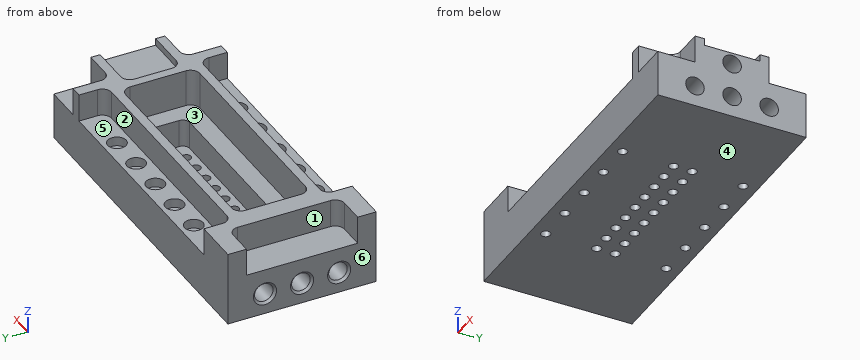
```python
from build123d import *

# Parameters (mm, degrees)
SKETCH1_W           = 230.1875
SKETCH1_H           = 101.6
BASE_EXTRUDE_DEPTH  = 50.8
CUT_EXTRUDE1_DEPTH  = 25.4
CUT_EXTRUDE2_DEPTH  = 19.05
CUT_EXTRUDE3_DEPTH  = 19.05
SKETCH5_R           = 6.35
CUT_EXTRUDE4_DEPTH  = 25.4
CHAMFER2_SIZE       = 1.5748
CUT_EXTRUDE5_START  = -25.4
SKETCH6_R           = 6.35
CUT_EXTRUDE5_DEPTH  = 25.4
CUT_EXTRUDE6_DEPTH  = 19.05
SKETCH8_R           = 3.175
CUT_EXTRUDE7_DEPTH  = 135.113217679
CUT_EXTRUDE8_DEPTH  = 19.05
SKETCH10_R          = 3.175
CUT_EXTRUDE9_DEPTH  = 131.455414438
SKETCH11_R          = 6.35
CUT_EXTRUDE10_DEPTH = 6.35
CUT_EXTRUDE11_DEPTH = 4.7498


with BuildPart() as part:
    # Sketch1 → Base-Extrude (new body)
    with BuildSketch(Plane.XY):
        with Locations((0.79375, 0)):
            Rectangle(SKETCH1_W, SKETCH1_H)
    extrude(amount=BASE_EXTRUDE_DEPTH)

    # Sketch2 → Cut-Extrude1 (cut)
    with BuildSketch(Plane.XY.offset(50.8)):
        with BuildLine():
            Line((-69.85, 25.4), (69.85, 25.4))
            ThreePointArc((69.85, 25.4), (74.340128061, 23.540128061), (76.2, 19.05))
            Line((76.2, 19.05), (76.2, -19.05))
            ThreePointArc((76.2, -19.05), (74.340128061, -23.540128061), (69.85, -25.4))
            Line((69.85, -25.4), (-69.85, -25.4))
            ThreePointArc((-69.85, -25.4), (-74.340128061, -23.540128061), (-76.2, -19.05))
            Line((-76.2, -19.05), (-76.2, 19.05))
            ThreePointArc((-76.2, 19.05), (-74.340128061, 23.540128061), (-69.85, 25.4))
        make_face()
    extrude(amount=-CUT_EXTRUDE1_DEPTH, mode=Mode.SUBTRACT)

    # Sketch3 → Cut-Extrude2 (cut)
    with BuildSketch(Plane.XY.offset(50.8)):
        with BuildLine():
            Line((136.525, 61.9125), (90.4875, 61.9125))
            Line((90.4875, 61.9125), (90.4875, 31.75))
            ThreePointArc((90.4875, 31.75), (92.347371939, 27.259871939), (96.8375, 25.4))
            Line((96.8375, 25.4), (136.525, 25.4))
            Line((136.525, 25.4), (136.525, 61.9125))
        make_face()
        with BuildLine():
            Line((136.525, -57.15), (90.4875, -57.15))
            Line((90.4875, -57.15), (90.4875, -31.75))
            ThreePointArc((90.4875, -31.75), (92.347371939, -27.259871939), (96.8375, -25.4))
            Line((96.8375, -25.4), (136.525, -25.4))
            Line((136.525, -25.4), (136.525, -57.15))
        make_face()
    extrude(amount=-CUT_EXTRUDE2_DEPTH, mode=Mode.SUBTRACT)

    # Sketch4 → Cut-Extrude3 (cut)
    with BuildSketch(Plane.XY.offset(50.8)):
        with BuildLine():
            Line((-120.65, 38.1), (-96.8375, 38.1))
            ThreePointArc((-96.8375, 38.1), (-92.347371939, 36.240128061), (-90.4875, 31.75))
            Line((-90.4875, 31.75), (-90.4875, -31.75))
            ThreePointArc((-90.4875, -31.75), (-92.347371939, -36.240128061), (-96.8375, -38.1))
            Line((-96.8375, -38.1), (-120.65, -38.1))
            Line((-120.65, -38.1), (-120.65, 38.1))
        make_face()
    extrude(amount=-CUT_EXTRUDE3_DEPTH, mode=Mode.SUBTRACT)

    # Sketch5 → Cut-Extrude4 (cut)
    with BuildSketch(Plane.ZY.offset(114.3)):
        with Locations((14.2875, 0)):
            Circle(SKETCH5_R)
        with Locations((14.2875, -25.4)):
            Circle(SKETCH5_R)
        with Locations((14.2875, 25.4)):
            Circle(SKETCH5_R)
    extrude(amount=-CUT_EXTRUDE4_DEPTH, mode=Mode.SUBTRACT)

    # Chamfer2
    chamfer2_edges = [part.edges().sort_by_distance(p)[0] for p in [
        (-114.3, -25.4, 7.9375),
        (-114.3, 0, 7.9375),
        (-114.3, 25.4, 7.9375),
    ]]
    chamfer(chamfer2_edges, length=CHAMFER2_SIZE)

    # Sketch6 → Cut-Extrude5 (cut)
    with BuildSketch(Plane(origin=(115.8875, 0, 0), x_dir=(0, 0, -1), z_dir=(1, 0, 0)).offset(CUT_EXTRUDE5_START)):
        with Locations((-38.1, 0)):
            Circle(SKETCH6_R)
        with Locations(Location((-14.2875, 0, 0), (0, 0, 180))):
            Circle(SKETCH6_R)
        with Locations(Location((-14.2875, 25.4, 0), (0, 0, 180))):
            Circle(SKETCH6_R)
        with Locations(Location((-14.2875, -25.4, 0), (0, 0, 180))):
            Circle(SKETCH6_R)
    extrude(amount=CUT_EXTRUDE5_DEPTH, mode=Mode.SUBTRACT)

    # Sketch7 → Cut-Extrude6 (cut)
    with BuildSketch(Plane.XY.offset(25.4)):
        with BuildLine():
            Line((-58.7375, 12.7), (58.7375, 12.7))
            ThreePointArc((58.7375, 12.7), (62.105096045, 11.305096045), (63.5, 7.9375))
            Line((63.5, 7.9375), (63.5, -7.9375))
            ThreePointArc((63.5, -7.9375), (62.105096045, -11.305096045), (58.7375, -12.7))
            Line((58.7375, -12.7), (-58.7375, -12.7))
            ThreePointArc((-58.7375, -12.7), (-62.105096045, -11.305096045), (-63.5, -7.9375))
            Line((-63.5, -7.9375), (-63.5, 7.9375))
            ThreePointArc((-63.5, 7.9375), (-62.105096045, 11.305096045), (-58.7375, 12.7))
        make_face()
    extrude(amount=-CUT_EXTRUDE6_DEPTH, mode=Mode.SUBTRACT)

    # Sketch8 → Cut-Extrude7 (cut, through all)
    with BuildSketch(Plane.XY.offset(6.35)):
        with Locations((-50.8, 6.35)):
            Circle(SKETCH8_R)
        with Locations((-38.1, 6.35)):
            Circle(SKETCH8_R)
        with Locations((-25.4, 6.35)):
            Circle(SKETCH8_R)
        with Locations((-12.7, 6.35)):
            Circle(SKETCH8_R)
        with Locations((0, 6.35)):
            Circle(SKETCH8_R)
        with Locations((12.7, 6.35)):
            Circle(SKETCH8_R)
        with Locations((25.4, 6.35)):
            Circle(SKETCH8_R)
        with Locations((38.1, 6.35)):
            Circle(SKETCH8_R)
        with Locations((50.8, 6.35)):
            Circle(SKETCH8_R)
        with Locations((-50.8, -6.35)):
            Circle(SKETCH8_R)
        with Locations((-38.1, -6.35)):
            Circle(SKETCH8_R)
        with Locations((-25.4, -6.35)):
            Circle(SKETCH8_R)
        with Locations((-12.7, -6.35)):
            Circle(SKETCH8_R)
        with Locations((0, -6.35)):
            Circle(SKETCH8_R)
        with Locations((12.7, -6.35)):
            Circle(SKETCH8_R)
        with Locations((25.4, -6.35)):
            Circle(SKETCH8_R)
        with Locations((38.1, -6.35)):
            Circle(SKETCH8_R)
        with Locations((50.8, -6.35)):
            Circle(SKETCH8_R)
    extrude(amount=-CUT_EXTRUDE7_DEPTH, mode=Mode.SUBTRACT)

    # Sketch9 → Cut-Extrude8 (cut)
    with BuildSketch(Plane.XY.offset(50.8)):
        with BuildLine():
            Line((-82.55, 63.5), (82.55, 63.5))
            Line((82.55, 63.5), (82.55, 38.1))
            ThreePointArc((82.55, 38.1), (80.690128061, 33.609871939), (76.2, 31.75))
            Line((76.2, 31.75), (-76.2, 31.75))
            ThreePointArc((-76.2, 31.75), (-80.690128061, 33.609871939), (-82.55, 38.1))
            Line((-82.55, 38.1), (-82.55, 63.5))
        make_face()
        with BuildLine():
            Line((-82.55, -60.325), (82.55, -60.325))
            Line((82.55, -60.325), (82.55, -38.1))
            ThreePointArc((82.55, -38.1), (80.690128061, -33.609871939), (76.2, -31.75))
            Line((76.2, -31.75), (-76.2, -31.75))
            ThreePointArc((-76.2, -31.75), (-80.690128061, -33.609871939), (-82.55, -38.1))
            Line((-82.55, -38.1), (-82.55, -60.325))
        make_face()
    extrude(amount=-CUT_EXTRUDE8_DEPTH, mode=Mode.SUBTRACT)

    # Sketch10 → Cut-Extrude9 (cut, through all)
    with BuildSketch(Plane.XY.offset(31.75)):
        with Locations((0, -41.275)):
            Circle(SKETCH10_R)
        with Locations((25.4, -41.275)):
            Circle(SKETCH10_R)
        with Locations((50.8, -41.275)):
            Circle(SKETCH10_R)
        with Locations((-25.4, -41.275)):
            Circle(SKETCH10_R)
        with Locations((-50.8, -41.275)):
            Circle(SKETCH10_R)
        with Locations((0, 41.275)):
            Circle(SKETCH10_R)
        with Locations((25.4, 41.275)):
            Circle(SKETCH10_R)
        with Locations((50.8, 41.275)):
            Circle(SKETCH10_R)
        with Locations((-25.4, 41.275)):
            Circle(SKETCH10_R)
        with Locations((-50.8, 41.275)):
            Circle(SKETCH10_R)
    extrude(amount=-CUT_EXTRUDE9_DEPTH, mode=Mode.SUBTRACT)

    # Sketch11 → Cut-Extrude10 (cut)
    with BuildSketch(Plane.XY.offset(31.75)):
        with Locations((-50.8, 41.275)):
            Circle(SKETCH11_R)
        with Locations((-25.4, 41.275)):
            Circle(SKETCH11_R)
        with Locations((0, 41.275)):
            Circle(SKETCH11_R)
        with Locations((25.4, 41.275)):
            Circle(SKETCH11_R)
        with Locations((50.8, 41.275)):
            Circle(SKETCH11_R)
        with Locations((-50.8, -41.275)):
            Circle(SKETCH11_R)
        with Locations((-25.4, -41.275)):
            Circle(SKETCH11_R)
        with Locations((0, -41.275)):
            Circle(SKETCH11_R)
        with Locations((25.4, -41.275)):
            Circle(SKETCH11_R)
        with Locations((50.8, -41.275)):
            Circle(SKETCH11_R)
    extrude(amount=-CUT_EXTRUDE10_DEPTH, mode=Mode.SUBTRACT)

    # Sketch12 → Cut-Extrude11 (cut)
    with BuildSketch(Plane.XY.offset(50.8)):
        with BuildLine():
            Line((88.9, 19.05), (123.825, 19.05))
            Line((123.825, 19.05), (123.825, -19.05))
            Line((123.825, -19.05), (88.9, -19.05))
            ThreePointArc((88.9, -19.05), (84.409871939, -17.190128061), (82.55, -12.7))
            Line((82.55, -12.7), (82.55, 12.7))
            ThreePointArc((82.55, 12.7), (84.409871939, 17.190128061), (88.9, 19.05))
        make_face()
    extrude(amount=-CUT_EXTRUDE11_DEPTH, mode=Mode.SUBTRACT)


solid = part.part
```
Part model, mm, in its own coordinate system. Face numbers are marked on the shaded views. A direction names the side the tool comes from. Give positions to 0.01 mm unless a question says otherwise; leave off trailing zeros. Write each loop counter-clockwise with the first axis right and the second up, starting at its lowest first coordinate (ties: lowest second). Pieces come first, ordered by that corner, then holes. Notation, with made-up numbers: (-22, 81.5) -> (19, 81.5) arc R14 cw to (19, 105.5) -> close; hole circle Ø9 at (-32.75, 67.25). An arc over 180 degrees is marked (long way). Put each result on its own line as item: value. Start each with the question number.
Item 1: Cut at A-A (x = 38.1). List the corners of the cut face in (y, z) (3 decimals).
Item 2: Pin check, flat tips, straight feed: pin 1 Ø11.5 at (x, y) = (0, -41.275) entering from +Z; pin 2 Ø5 at (y, z) = (3, 12.5) entering from -X; pin 3 Ø5 at (x, z) = (22, 38) entering from -Y. Stop position of each tip, or through.
Item 3: Which spindle directions (+Z, -Z, +X, -X, +Y, -Y) get a long thin tool onto all of the face, cutting with end or side? Do the marked faces 1, 2 and 3. Say none if no direction does.
Item 4: Pull direction X, two halves, no side cores. Call the marked faces 4, 5 and 6: pulls with the +X half, pulls with the -X half, needs draft (parallel to the pull), parting line crosses it, or undercut.
Item 5: Wall check: L1, parallel to Y at x = 50.8, z = 8.25; L2, parallel to Y at x = -50.8, z = 2.25 (3 decimals); L3, parallel to Y at x = 25.4, z = 27.25 (3 decimals). Give the ranges that are in metal, low to high. Write a range as [from, to].
Item 6: Cut at C-C (x = -94). List the corners of the cut face in (y, z), then the cut area to 3 significant figures.
Item 7: Cut at D-D (x = 79). List the corners of the cut face in (y, z).
Answer list:
1. outline: (-50.8, 0) -> (-9.525, 0) -> (-9.525, 6.35) -> (-12.7, 6.35) -> (-12.7, 25.4) -> (-25.4, 25.4) -> (-25.4, 50.8) -> (-31.75, 50.8) -> (-31.75, 31.75) -> (-50.8, 31.75) -> close; (-3.175, 0) -> (3.175, 0) -> (3.175, 6.35) -> (-3.175, 6.35) -> close; (9.525, 0) -> (50.8, 0) -> (50.8, 31.75) -> (31.75, 31.75) -> (31.75, 50.8) -> (25.4, 50.8) -> (25.4, 25.4) -> (12.7, 25.4) -> (12.7, 6.35) -> (9.525, 6.35) -> close
2. pin 1: stops at z = 25.4
2. pin 2: stops at x = -88.9
2. pin 3: stops at y = -31.75
3. face 1: +Z, -X
3. face 2: +Z, +Y
3. face 3: +Z
4. face 4: needs draft
4. face 5: undercut
4. face 6: pulls with the -X half
5. L1: y = [-50.8, -44.45], [-38.1, -12.7], [12.7, 38.1], [44.45, 50.8]
5. L2: y = [-50.8, -44.45], [-38.1, -9.525], [-3.175, 3.175], [9.525, 38.1], [44.45, 50.8]
5. L3: y = [-50.8, -47.625], [-34.925, -25.4], [25.4, 34.925], [47.625, 50.8]
6. outline: (-50.8, 0) -> (50.8, 0) -> (50.8, 50.8) -> (37.43, 50.8) -> (37.43, 31.75) -> (-37.43, 31.75) -> (-37.43, 50.8) -> (-50.8, 50.8) -> close; hole circle Ø12.7 at (-25.4, 14.29); hole circle Ø12.7 at (0, 14.29); hole circle Ø12.7 at (25.4, 14.29)
6. area: 3,360 mm2
7. outline: (-50.8, 0) -> (50.8, 0) -> (50.8, 31.75) -> (32.4, 31.75) -> (32.4, 50.8) -> (-32.4, 50.8) -> (-32.4, 31.75) -> (-50.8, 31.75) -> close
